Build history of the part. All positions in model axes, mm. A direction names the side the tool comes from. Give positions to 0.01 mm unless a question says otherwise; leave off trailing zeros. Order: outer loops, then holes, each group sorted by start corner. A loop starts at its lowest first (then second) coordinate and runs counter-clockwise, first axis right, second up. Notation, with made-up numbers: M 37.25,41 L 76.25,41 A21 ccw 76.25,63 Z; hole C 37.5,-13 d1. An arc over 180 degrees is marked long. One line per item, written item: value. Start each with the question number.
from build123d import *

# Parameters (mm, degrees)
SKETCH_1_W              = 52
SKETCH_1_H              = 52
EXTRUDE_1_DEPTH         = 31
SKETCH_2_W              = 20.5
SKETCH_2_H              = 52
CUT_EXTRUDE_1_DEPTH     = 20
SKETCH_5_R              = 26
EXTRUDE_2_DEPTH         = 31
CUT_EXTRUDE_2_DEPTH     = 32
SKETCH_7_W              = 20
SKETCH_7_H              = 20.5
CUT_EXTRUDE_3_DEPTH     = 53
EXTRUDE_3_DEPTH         = 27
SKETCH_10_W             = 19
SKETCH_10_H             = 14
SKETCH_11_W             = 19
SKETCH_11_H             = 28
CUT_EXTRUDE_4_DEPTH     = 27
EXTRUDE_4_DEPTH         = 52
SKETCH_13_R             = 2.1
CUT_EXTRUDE_5_DEPTH     = 59
SKETCH_14_R             = 2.1
CUT_EXTRUDE_6_DEPTH     = 48.25
SKETCH_15_R             = 5
CUT_EXTRUDE_7_DEPTH     = 43.2500001
SKETCH_17_W             = 10
SKETCH_17_H             = 42.25
CUT_EXTRUDE_8_DEPTH     = 6.0000001
SKETCH_18_R             = 5
CUT_EXTRUDE_9_DEPTH     = 28.0000001
SKETCH_19_R             = 2.5
CUT_EXTRUDE_10_DEPTH    = 59.0000001
CUT_EXTRUDE1_DEPTH      = 53.0000001
SKETCH3_R               = 7.5
CUT_EXTRUDE2_DEPTH      = 22.300523217
CUT_EXTRUDE2_DEPTH_BACK = 2
CUT_EXTRUDE_11_DEPTH    = 28.0000001
SKETCH_21_W             = 15
SKETCH_21_H             = 9.144379334
EXTRUDE_5_DEPTH         = 21
CUT_EXTRUDE_12_DEPTH    = 15
FILLET_1_R              = 3


with BuildPart() as part:
    # Эскиз1 → Бобышка-Вытянуть1 (new body)
    with BuildSketch(Plane.XY):
        with Locations((26, 0)):
            Rectangle(SKETCH_1_W, SKETCH_1_H)
    extrude(amount=EXTRUDE_1_DEPTH)

    # Эскиз2 → Вырез-Вытянуть1 (cut)
    with BuildSketch(Plane.ZY):
        with Locations((15.5, 0)):
            Rectangle(SKETCH_2_W, SKETCH_2_H)
    extrude(amount=-CUT_EXTRUDE_1_DEPTH, mode=Mode.SUBTRACT)

    # Эскиз5 → Бобышка-Вытянуть2 (add)
    with BuildSketch(Plane.XY.offset(31)):
        with Locations((41.25, 0)):
            Circle(SKETCH_5_R)
    extrude(amount=-EXTRUDE_2_DEPTH)

    # Эскиз6 → Вырез-Вытянуть2 (cut, through all)
    with BuildSketch(Plane.XY.offset(31)):
        with BuildLine():
            Line((52, 23.673561202), (52, 26))
            Line((52, 26), (25, 26))
            ThreePointArc((25, 26), (38.550021379, 25.417314778), (52, 23.673561202))
        make_face()
    cut_extrude_2 = extrude(amount=-CUT_EXTRUDE_2_DEPTH, mode=Mode.SUBTRACT)

    # Зеркальное отражение1: Вырез-Вытянуть2 across plane
    add(cut_extrude_2.mirror(Plane(origin=(0, 0, 0), x_dir=(0, 0, 1), z_dir=(0, -1, 0))), mode=Mode.SUBTRACT)

    # Эскиз7 → Вырез-Вытянуть3 (cut, through all)
    with BuildSketch(Plane(origin=(0, 26, 0), x_dir=(1, 0, 0), z_dir=(0, 1, 0))):
        with Locations((10, -15.5)):
            Rectangle(SKETCH_7_W, SKETCH_7_H)
    extrude(amount=-CUT_EXTRUDE_3_DEPTH, mode=Mode.SUBTRACT)

    # Эскиз9 → Бобышка-Вытянуть3 (add)
    with BuildSketch(Plane(origin=(0, 0, 0), x_dir=(-1, 0, 0), z_dir=(0, 0, -1))):
        with BuildLine():
            Line((-25, 26), (-25, -26))
            ThreePointArc((-25, -26), (-38.550021379, -25.417314778), (-52, -23.673561202))
            ThreePointArc((-52, -23.673561202), (-67.25, 0), (-52, 23.673561202))
            ThreePointArc((-52, 23.673561202), (-38.550021379, 25.417314778), (-25, 26))
        make_face()
    extrude(amount=EXTRUDE_3_DEPTH)

    # Эскиз10 → Вырез-Повернуть2 (revolve, cut)
    with BuildSketch(Plane.ZY.offset(-41.25)):
        with Locations((-11.25, 7)):
            Rectangle(SKETCH_10_W, SKETCH_10_H)
    revolve(axis=Axis((41.25, 0, -20.75), (0, 0, 1)), mode=Mode.SUBTRACT)

    # Эскиз11 → Вырез-Вытянуть4 (cut, through all)
    with BuildSketch(Plane(origin=(0, 0, 0), x_dir=(0, 0, -1), z_dir=(0, -1, 0))):
        with Locations((11.25, 41.25)):
            Rectangle(SKETCH_11_W, SKETCH_11_H)
    extrude(amount=CUT_EXTRUDE_4_DEPTH, mode=Mode.SUBTRACT)

    # Эскиз12 → Бобышка-Вытянуть4 (add)
    with BuildSketch(Plane.XZ.offset(26)):
        with BuildLine():
            Line((0, 0), (25, 0))
            Line((25, 0), (25, -27))
            ThreePointArc((25, -27), (16.039335617, -10.222837391), (0, 0))
        make_face()
    extrude(amount=-EXTRUDE_4_DEPTH)

    # Эскиз13 → Вырез-Вытянуть5 (cut, through all)
    with BuildSketch(Plane.XY.offset(31)):
        with Locations((10, 0)):
            Circle(SKETCH_13_R)
    extrude(amount=-CUT_EXTRUDE_5_DEPTH, mode=Mode.SUBTRACT)

    # Эскиз14 → Вырез-Вытянуть6 (cut, through all)
    with BuildSketch(Plane.ZY.offset(-20)):
        with Locations((15.5, -21)):
            Circle(SKETCH_14_R)
        with Locations((15.5, 21)):
            Circle(SKETCH_14_R)
    extrude(amount=-CUT_EXTRUDE_6_DEPTH, mode=Mode.SUBTRACT)

    # Эскиз15 → Вырез-Вытянуть7 (cut, through all)
    with BuildSketch(Plane(origin=(25, 0, 0), x_dir=(0, 0, -1), z_dir=(1, 0, 0))):
        with Locations((-15.5, 21)):
            Circle(SKETCH_15_R)
        with Locations((-15.5, -21)):
            Circle(SKETCH_15_R)
    extrude(amount=CUT_EXTRUDE_7_DEPTH, mode=Mode.SUBTRACT)

    # Эскиз17 → Вырез-Вытянуть8 (cut, through all)
    with BuildSketch(Plane(origin=(0, 21, 0), x_dir=(0, 0, -1), z_dir=(0, 1, 0))):
        with Locations((-15.5, -46.125)):
            Rectangle(SKETCH_17_W, SKETCH_17_H)
    cut_extrude_8 = extrude(amount=CUT_EXTRUDE_8_DEPTH, mode=Mode.SUBTRACT)

    # Зеркальное отражение2: Вырез-Вытянуть8 across plane
    add(cut_extrude_8.mirror(Plane(origin=(0, 0, 0), x_dir=(0, 0, 1), z_dir=(0, -1, 0))), mode=Mode.SUBTRACT)

    # Эскиз18 → Вырез-Вытянуть9 (cut, through all)
    with BuildSketch(Plane(origin=(0, 0, 0), x_dir=(-1, 0, 0), z_dir=(0, 0, -1))):
        with Locations((-10, 0)):
            Circle(SKETCH_18_R)
    extrude(amount=CUT_EXTRUDE_9_DEPTH, mode=Mode.SUBTRACT)

    # Эскиз19 → Вырез-Вытянуть10 (cut, through all)
    with BuildSketch(Plane.XY.offset(31)):
        with Locations((41.25, 0)):
            Circle(SKETCH_19_R)
    extrude(amount=-CUT_EXTRUDE_10_DEPTH, mode=Mode.SUBTRACT)

    # Sketch1 → Cut-Extrude1 (cut, through all)
    with BuildSketch(Plane(origin=(0, 26, 0), x_dir=(1, 0, 0), z_dir=(0, 1, 0))):
        with BuildLine():
            Line((25, -31), (67.25, -31))
            Line((67.25, -31), (67.25, -3.25))
            ThreePointArc((67.25, -3.25), (41.975877859, -10.807868092), (25, -31))
        make_face()
    extrude(amount=-CUT_EXTRUDE1_DEPTH, mode=Mode.SUBTRACT)

    # Sketch3 → Cut-Extrude2 (cut, two sides)
    with BuildSketch(Plane.XY.offset(9.699476883)) as cut_extrude2_sk:
        with Locations((41.25, 0)):
            Circle(SKETCH3_R)
    extrude(amount=CUT_EXTRUDE2_DEPTH, mode=Mode.SUBTRACT)
    extrude(cut_extrude2_sk.sketch, amount=-CUT_EXTRUDE2_DEPTH_BACK, mode=Mode.SUBTRACT)

    # Эскиз20 → Вырез-Вытянуть11 (cut, through all)
    with BuildSketch(Plane(origin=(0, 0, 0), x_dir=(-1, 0, 0), z_dir=(0, 0, -1))):
        with BuildLine():
            Line((-10, 5), (0, 5))
            Line((0, 5), (0, -5))
            Line((0, -5), (-15, -5))
            Line((-15, -5), (-15, 0))
            ThreePointArc((-15, 0), (-13.535533906, 3.535533906), (-10, 5))
        make_face()
    extrude(amount=CUT_EXTRUDE_11_DEPTH, mode=Mode.SUBTRACT)

    # Эскиз21 → Бобышка-Вытянуть5 (add)
    with BuildSketch(Plane(origin=(0, -5, 0), x_dir=(1, 0, 0), z_dir=(0, 1, 0))):
        with Locations((7.5, 4.572189667)):
            Rectangle(SKETCH_21_W, SKETCH_21_H)
    extrude(amount=-EXTRUDE_5_DEPTH)

    # Эскиз22 → Вырез-Вытянуть12 (cut)
    with BuildSketch(Plane.XZ.offset(26)):
        Polygon((10, 1.925426481), (7.25, 0.33771324), (7.25, -2.83771324), (10, -4.425426481), (12.75, -2.83771324), (12.75, 0.33771324), align=None)
    extrude(amount=-CUT_EXTRUDE_12_DEPTH, mode=Mode.SUBTRACT)

    # Скругление1
    fillet_1_edges = [part.edges().sort_by_distance(p)[0] for p in [
        (0, -15.5, -9.144379334),
    ]]
    fillet(fillet_1_edges, radius=FILLET_1_R)


solid = part.part
1) Drill centre lines: line 1 (Y direction, x = 23.2, z = 15.5); line 2 (Z direction, x = 4.5, y = -15); line 3 (Y direction, x = 10, z = 3.25). Where is each one in solid material? Low to high.
2) Drop flat-ended pins along their axis: P1, Ø4, axis at y = -2, z = -5, coming from the -X side; P2, Ø5.5, axis at x = 33, y = 24, coming from the +Z side; P3, Ø6, axis at x = 11.5, y = -10.5, coming from the -Z side. Give the stop position or say it passes through.
3) Pull direction Y, two halves, no side cores. Call faces 6 (the flat face through (15, -26, 2)), 7 (the flat face through (41, -6, -20.75)), 8 (the cylindrical face through (43.56, -0.96, -23.83)): pulls with the +Y half, pulls with the -Y half, needs draft (parallel to the pull), parting line crosses it, or undercut.
4) Slice it at C-C (x = 46). List the corners of the cut face in (y, z), plus the area to 3 significant figures.
5) Slice it at D-D (z = -12.5). List the corners of the cut face in (x, y), plus the area to 3 significant figures.
6) Tool access for faces 1 (the flat face through (7, -5, -5)), 2 (the cylindrical face through (26.71, -25.99, 23.49)), 3 (the flat face through (25, -23, 14)), 4 (the flat face through (8.606, -18.605, -3.62)), 5 (the flat face through (20, 0, 15)): list every direction of +Z, -Z, +X, -X, +Y, -Y with a clear straight run to the whole face (end or side of a thin tool).
7) Slice it at A-A (z = 27). List the corners of the cut face in (x, y), plus the area to 3 significant figures.
8) Slice it at B-B (z = 15.5). List the corners of the cut face in (x, y).
Results list:
1. line 1: y = -26 to -23.1, -18.9 to 18.9, 23.1 to 26
1. line 2: z = -9.14 to 5.25, 25.75 to 31
1. line 3: y = -26 to -2.1, 2.1 to 26
2. P1: stops at x = 15
2. P2: stops at z = 21.89
2. P3: stops at z = -9.14
3. face 6: pulls with the -Y half
3. face 7: needs draft
3. face 8: undercut
4. outline: M -24.6,-27 L 24.6,-27 L 24.6,8.45 L 5.8,8.45 L 5.8,7.7 L -5.8,7.7 L -5.8,8.45 L -24.6,8.45 L -24.6,-1.75 L 13.17,-1.75 L 13.17,-20.75 L -24.6,-20.75 Z
4. area: 1,020 mm²
5. outline: M 17.98,-26 L 25,-26 A157.84 ccw 27.25,-25.98 L 27.25,0 A14 cw 55.25,0 L 55.25,-21.91 A26 ccw 52,23.67 A157.84 ccw 25,26 L 17.98,26 Z
5. area: 1,240 mm²
6. face 1: -Z, -X
6. face 2: +Z, -Z, +X, -Y
6. face 3: +X, -Y
6. face 4: -Y
6. face 5: -X, +Y, -Y
7. outline: M 0,-26 L 25,-26 A157.84 ccw 26.97,-25.99 L 26.97,25.99 A157.84 ccw 25,26 L 0,26 Z; hole C 10,0 d4.2
7. area: 1,390 mm²
8. outline: M 20,-26 L 25,-26 L 25,-23.1 L 20,-23.1 Z; M 20,-18.9 L 25,-18.9 L 25,-16 L 35.98,-16 L 35.98,-5.34 A7.5 cw 35.98,5.34 L 35.98,16 L 25,16 L 25,18.9 L 20,18.9 Z; M 20,23.1 L 25,23.1 L 25,26 L 20,26 Z
